Can you work these out from the model? Positions are in its coordinate system, mm. A direction names the side the tool comes from. Give positions to 0.01 mm unless a question says otherwise; leave off trailing zeros.
Autodesk Inventor part; units mm, degrees
ref_plane "YZ Plane" through (0, 0, 0) normal (1, 0, 0) x (0, 1, 0)
ref_plane "XZ Plane" through (0, 0, 0) normal (0, 1, 0) x (-1, 0, 0)
ref_plane "XY Plane" through (0, 0, 0) normal (0, 0, 1) x (1, 0, 0)
sketch "스케치1" plane through (0, 0, 0) normal (0, 1, 0) x (-1, 0, 0)
  point P0 (0, 0)
sketch "스케치2" plane through (0, 0, 0) normal (0, 1, 0) x (-1, 0, 0)
  line L0 (10, 0) -> (167.5, 0)
  line L1 (177.5, -10) -> (177.5, -239.5)
  line L2 (167.5, -249.5) -> (10, -249.5)
  line L3 (0, -239.5) -> (0, -10)
  arc A0 (177.5, -10) -> (167.5, 0) centre (167.5, -10) ccw
  arc A1 (10, 0) -> (0, -10) centre (10, -10) ccw
  arc A2 (0, -239.5) -> (10, -249.5) centre (10, -239.5) ccw
  arc A3 (167.5, -249.5) -> (177.5, -239.5) centre (167.5, -239.5) ccw
  point P0 (0, 0)
  point P1 (177.5, -249.5)
  point P2 (177.5, 0)
  point P3 (0, -249.5)
  dimension "d19" = 177.5
  dimension "d20" = 249.5
  dimension "d21" = 10
extrude "돌출1" add sketch "스케치2" along normal blind 5.3
fillet "모깎기1" radius 0.6 8 edges at (-2.9289, 5.3, -246.5711) (-88.75, 5.3, -249.5) (-174.5711, 5.3, -246.5711) (-177.5, 5.3, -124.75) (-174.5711, 5.3, -2.9289) (-88.75, 5.3, 0) (-2.9289, 5.3, -2.9289) (0, 5.3, -124.75)
fillet "모깎기2" radius 0.6 8 edges at (-2.9289, 0, -246.5711) (-88.75, 0, -249.5) (-174.5711, 0, -246.5711) (-177.5, 0, -124.75) (-174.5711, 0, -2.9289) (-88.75, 0, 0) (-2.9289, 0, -2.9289) (0, 0, -124.75)
sketch "스케치3" plane through (-167.5, 4.7, 0) normal (0, 0, 1) x (1, 0, 0)
  line L0 (0, -4.1) -> (0, 0)
  line L1 (11, -2.05) -> (11, -1.05)
  line L2 (11, -2.05) -> (11, -2.05)
  line L3 (12, -3.05) -> (20, -3.05)
  line L4 (21, -2.05) -> (21, -2.05)
  line L5 (20, -1.05) -> (12, -1.05)
  arc A0 (12, -1.05) -> (11, -2.05) centre (12, -2.05) ccw
  arc A1 (11, -2.05) -> (12, -3.05) centre (12, -2.05) ccw
  arc A2 (20, -3.05) -> (21, -2.05) centre (20, -2.05) ccw
  arc A3 (21, -2.05) -> (20, -1.05) centre (20, -2.05) ccw
  point P0 (167.5, -4.7)
  point P1 (11, -3.05)
  point P2 (21, -3.05)
  point P3 (11, -2.05)
  point P4 (21, -2.05)
  dimension "d29" = 10
  dimension "d30" = 1
extrude "돌출2" add sketch "스케치3" along normal blind 0.5
sketch "스케치4" plane through (0, 5.3, 0) normal (0, 1, 0) x (1, 0, 0)
  line L0 (-176.9, 239.5) -> (-176.9, 10)
  line L1 (-0.6, 239.5) -> (-0.6, 10)
  line L2 (-164.5, 10) -> (-13, 10)
  arc A0 (-176.9, 10) -> (-167.5, 0.6) centre (-167.5, 10) ccw
  arc A1 (-167.5, 248.9) -> (-176.9, 239.5) centre (-167.5, 239.5) ccw
  line L3 (-167.5, 13) -> (-167.5, 236.5)
  line L4 (-164.5, 239.5) -> (-13, 239.5)
  line L5 (-167.5, 248.9) -> (-10, 248.9)
  line L6 (-10, 236.5) -> (-10, 13)
  arc A2 (-164.5, 239.5) -> (-167.5, 236.5) centre (-164.5, 236.5) ccw
  arc A3 (-10, 236.5) -> (-13, 239.5) centre (-13, 236.5) ccw
  arc A4 (-167.5, 13) -> (-164.5, 10) centre (-164.5, 13) ccw
  arc A5 (-13, 10) -> (-10, 13) centre (-13, 13) ccw
  point P0 (0, 0)
  dimension "d33" = 3
extrude "돌출3" cut sketch "스케치4" against normal blind 0.02
sketch "스케치5" plane through (0, 0, 0) normal (0, -1, 0) x (1, 0, 0)
  arc A0 (-167.5, -0.6) -> (-176.9, -10) centre (-167.5, -10) ccw
  line L0 (-165.85, -7.65) -> (-154.6582, -7.65)
  line L1 (-149.85, -12.4582) -> (-149.85, -22.8418)
  line L2 (-154.6582, -27.65) -> (-165.85, -27.65)
  line L3 (-170.6582, -22.8418) -> (-170.6582, -12.4582)
  arc A1 (-154.6582, -27.65) -> (-149.85, -22.8418) centre (-154.6582, -22.8418) ccw
  arc A2 (-149.85, -12.4582) -> (-154.6582, -7.65) centre (-154.6582, -12.4582) ccw
  arc A3 (-165.85, -7.65) -> (-170.6582, -12.4582) centre (-165.85, -12.4582) ccw
  arc A4 (-170.6582, -22.8418) -> (-165.85, -27.65) centre (-165.85, -22.8418) ccw
  circle A5 centre (-165.85, -12.4582) radius 2.75
  circle A6 centre (-165.85, -22.8418) radius 2.75
  line L4 (-154.6582, -22.8418) -> (-154.6582, -12.4582)
  circle A7 centre (-154.6582, -17.65) radius 2.4059
  point P0 (0, 0)
  dimension "d42" = 5.5
  dimension "d43" = 5.5
extrude "돌출4" add sketch "스케치5" along normal blind 0.5
sketch "스케치6" plane through (-154.6582, 0, -17.65) normal (0, -1, 0) x (1, 0, 0)
  circle A0 centre (0, 0) radius 2.4059
  point P0 (154.6582, 17.65)
extrude "돌출5" add sketch "스케치6" along normal blind 0.3
sketch "스케치7" plane through (-165.85, 0, -22.8418) normal (0, -1, 0) x (1, 0, 0)
  circle A0 centre (0, 0) radius 2.75
  point P0 (165.85, 22.8418)
extrude "돌출6" add sketch "스케치7" along normal blind 0.7
sketch "스케치8" plane through (-165.85, 0, -12.4582) normal (0, -1, 0) x (1, 0, 0)
  circle A0 centre (0, 0) radius 2.75
  point P0 (165.85, 12.4582)
extrude "돌출7" add sketch "스케치8" along normal blind 0.7
sketch "스케치9" plane through (-165.85, -0.7, -22.8418) normal (0, -1, 0) x (1, 0, 0)
  circle A0 centre (0, 0) radius 2.25
  point P0 (165.85, 22.8418)
  dimension "d52" = 4.5
extrude "돌출8" cut sketch "스케치9" against normal blind 0.1
sketch "스케치10" plane through (-165.85, -0.7, -12.4582) normal (0, -1, 0) x (1, 0, 0)
  circle A0 centre (0, 0) radius 2.25
  point P0 (165.85, 12.4582)
  dimension "d55" = 4.5
extrude "돌출9" cut sketch "스케치10" against normal blind 0.1
sketch "스케치11" plane through (-10, 4.7, -249.5) normal (0, 0, -1) x (-1, 0, 0)
  line L0 (0, -4.1) -> (0, 0)
  line L1 (157.5, -4.1) -> (157.5, 0)
  line L2 (77.75, -3.05) -> (81.75, -3.05)
  line L3 (81.75, -3.05) -> (75.75, -3.05)
  line L4 (74.75, -2.05) -> (74.75, -2.05)
  line L5 (75.75, -1.05) -> (81.75, -1.05)
  line L6 (82.75, -2.05) -> (82.75, -2.05)
  line L7 (0, -2.05) -> (74.75, -2.05)
  line L8 (82.75, -2.05) -> (157.5, -2.05)
  arc A0 (75.75, -1.05) -> (74.75, -2.05) centre (75.75, -2.05) ccw
  arc A1 (74.75, -2.05) -> (75.75, -3.05) centre (75.75, -2.05) ccw
  arc A2 (81.75, -3.05) -> (82.75, -2.05) centre (81.75, -2.05) ccw
  arc A3 (82.75, -2.05) -> (81.75, -1.05) centre (81.75, -2.05) ccw
  point P0 (-10, -4.7)
  point P1 (74.75, -2.05)
extrude "돌출10" cut sketch "스케치11" against normal blind 8
sketch "스케치12" plane through (-10, 4.7, -241.5) normal (0, 0, -1) x (-1, 0, 0)
  arc A0 (75.75, -1.05) -> (75.75, -3.05) centre (75.75, -2.05) ccw
  line L0 (75.75, -1.05) -> (81.75, -1.05)
  line L1 (76.75, -2.05) -> (76.75, -1.95)
  line L2 (0, -4.1) -> (157.5, -4.1)
  line L3 (76.85, -1.85) -> (80.65, -1.85)
  line L4 (80.75, -1.95) -> (80.75, -2.15)
  line L5 (80.65, -2.25) -> (76.85, -2.25)
  line L6 (76.75, -2.15) -> (76.75, -2.05)
  arc A1 (80.75, -1.95) -> (80.65, -1.85) centre (80.65, -1.95) ccw
  arc A2 (80.65, -2.25) -> (80.75, -2.15) centre (80.65, -2.15) ccw
  arc A3 (76.75, -2.15) -> (76.85, -2.25) centre (76.85, -2.15) ccw
  arc A4 (76.85, -1.85) -> (76.75, -1.95) centre (76.85, -1.95) ccw
  point P0 (-10, -4.7)
extrude "돌출11" add sketch "스케치12" along normal blind 6
sketch "스케치13" plane through (-10, 4.7, -249.5) normal (0, 0, -1) x (-1, 0, 0)
  line L0 (74.4634, -2.2843) -> (39.4634, -2.2843)
  circle A0 centre (39.4634, -2.2843) radius 0.75
  circle A1 centre (37.4634, -2.2843) radius 0.75
  circle A2 centre (35.4634, -2.2843) radius 0.75
  circle A3 centre (33.4634, -2.2843) radius 0.75
  circle A4 centre (31.4634, -2.2843) radius 0.75
  circle A5 centre (29.4634, -2.2843) radius 0.75
  circle A6 centre (27.4634, -2.2843) radius 0.75
  circle A7 centre (25.4634, -2.2843) radius 0.75
  circle A8 centre (23.4634, -2.2843) radius 0.75
  circle A9 centre (21.4634, -2.2843) radius 0.75
  circle A10 centre (19.4634, -2.2843) radius 0.75
  point P0 (-10, -4.7)
  dimension "d73" = 35
  dimension "d84" = 1.5
extrude "돌출12" cut sketch "스케치13" against normal blind 6
sketch "스케치14" plane through (-10, 4.7, -249.5) normal (0, 0, -1) x (-1, 0, 0)
  arc A0 (81.75, -3.05) -> (81.75, -1.05) centre (81.75, -2.05) ccw
  circle A1 centre (117.75, -2.05) radius 0.75
  circle A2 centre (119.75, -2.05) radius 0.75
  circle A3 centre (121.75, -2.05) radius 0.75
  circle A4 centre (123.75, -2.05) radius 0.75
  circle A5 centre (125.75, -2.05) radius 0.75
  circle A6 centre (127.75, -2.05) radius 0.75
  circle A7 centre (129.75, -2.05) radius 0.75
  circle A8 centre (137.75, -2.05) radius 0.75
  circle A9 centre (135.75, -2.05) radius 0.75
  circle A10 centre (133.75, -2.05) radius 0.75
  circle A11 centre (131.75, -2.05) radius 0.77
  point P0 (-10, -4.7)
extrude "돌출13" cut sketch "스케치14" against normal blind 6
fillet "모깎기3" radius 0.3 8 edges at (-169.2499, 0, -9.0583) (-160.2541, 0, -7.65) (-151.2583, 0, -9.0583) (-149.85, 0, -17.65) (-151.2583, 0, -26.2417) (-160.2541, 0, -27.65) (-169.2499, 0, -26.2417) (-170.6582, 0, -17.65)
properties part number "ipad"
(1) Thinking about a two-plate mould opening in X: for faces 1 (the cylindrical face through (-3.01, 2.62, -246.65)), 2 (the flat face through (-88, 0, -123)), 3 (the flat face through (-155, -0.3, -18)), 4 (the flat face through (-89, 3.65, -246)), which applies, pulls with the +X half, pulls with the -X half, needs draft (parallel to the pull), parting line crosses it, or undercut?
Returned:
face 1: pulls with the +X half
face 2: needs draft
face 3: undercut
face 4: undercut
(2) Which directions (+Z, -Z, +X, -X, +Y, -Y) give clear straight access to the entire face, cutting with the end or side of a thin tool? Please do faces 5 (the flat face through (-89, 1.65, -246)), 6 (the flat face through (-90, 5.28, -126)).
Returned:
face 5: -Z
face 6: +Z, -Z, +X, -X, +Y
(3) Will these pins go through, and if not, where does the flat tip stop? P1, Ø1.2, axis at x = -35.5, y = 3, coming from the -Z side; P2, Ø1.4, axis at x = -49.46, y = 2.42, coming from the +Z side; P3, Ø1.5, axis at x = -91.5, z = -125.5, coming from the +Y side; P4, Ø1.5, axis at x = -152, z = -85, coming from the -Y side.
Returned:
P1: stops at z = -249.5
P2: stops at z = 0
P3: stops at y = 5.28
P4: stops at y = 0
(4) Please list where these lines run through material, in increasing order: probe 1 along X at (y, z) = (-0.45, -17.65); probe 2 along Z at (x, y) = (-29, 1.7); probe 3 along Z at (x, y) = (-39, 2.9).
Returned:
probe 1: x = -170.66 to -157.06, -152.25 to -149.85
probe 2: z = -249.5 to 0
probe 3: z = -243.5 to 0
